```python
from build123d import *

# Parameters (mm, degrees)
BOSS_EXTRUDE1_DEPTH = 13
BOSS_EXTRUDE2_DEPTH = 2.5
SKETCH3_R           = 7
BOSS_EXTRUDE3_DEPTH = 5


with BuildPart() as part:
    # Sketch1 → Boss-Extrude1 (new body)
    with BuildSketch(Plane(origin=(0, 0, 0), x_dir=(1, 0, 0), z_dir=(0, 1, 0))):
        with BuildLine():
            ThreePointArc((5.85, 0), (5.148142373, 2.778332254), (3.210981158, 4.89))
            Line((3.210981158, 4.89), (-3.210981158, 4.89))
            ThreePointArc((-3.210981158, 4.89), (-5.148142373, 2.778332254), (-5.85, 0))
            Line((-5.85, 0), (5.85, 0))
        make_face()
        with BuildLine():
            ThreePointArc((3.210981158, -4.89), (5.148142373, -2.778332254), (5.85, 0))
            Line((5.85, 0), (-5.85, 0))
            ThreePointArc((-5.85, 0), (-5.148142373, -2.778332254), (-3.210981158, -4.89))
            Line((-3.210981158, -4.89), (3.210981158, -4.89))
        make_face()
    extrude(amount=BOSS_EXTRUDE1_DEPTH)

    # Sketch2 → Boss-Extrude2 (add)
    with BuildSketch(Plane(origin=(0, 13, 0), x_dir=(1, 0, 0), z_dir=(0, 1, 0))):
        with BuildLine():
            Line((0, 4.89), (0, 7.75))
            ThreePointArc((0, 7.75), (-4.510404638, 6.302281333), (-7.335700376, 2.5))
            ThreePointArc((-7.335700376, 2.5), (-7.75, 0), (-7.335700376, -2.5))
            ThreePointArc((-7.335700376, -2.5), (-4.510404638, -6.302281333), (0, -7.75))
            Line((0, -7.75), (0, -4.89))
            Line((0, -4.89), (-3.210981158, -4.89))
            ThreePointArc((-3.210981158, -4.89), (-5.85, 0), (-3.210981158, 4.89))
            Line((-3.210981158, 4.89), (0, 4.89))
        make_face()
        with BuildLine():
            ThreePointArc((7.335700376, 2.5), (4.510404638, 6.302281333), (0, 7.75))
            Line((0, 7.75), (0, 4.89))
            Line((0, 4.89), (3.210981158, 4.89))
            ThreePointArc((3.210981158, 4.89), (5.85, 0), (3.210981158, -4.89))
            Line((3.210981158, -4.89), (0, -4.89))
            Line((0, -4.89), (0, -7.75))
            ThreePointArc((0, -7.75), (4.510404638, -6.302281333), (7.335700376, -2.5))
            ThreePointArc((7.335700376, -2.5), (7.645723573, -1.267048162), (7.75, 0))
            ThreePointArc((7.75, 0), (7.645723573, 1.267048162), (7.335700376, 2.5))
        make_face()
        with BuildLine():
            Line((3.210981158, 4.89), (0, 4.89))
            Line((0, 4.89), (0, -4.89))
            Line((0, -4.89), (3.210981158, -4.89))
            ThreePointArc((3.210981158, -4.89), (5.85, 0), (3.210981158, 4.89))
        make_face()
        with BuildLine():
            Line((9.835700376, 2.5), (7.335700376, 2.5))
            ThreePointArc((7.335700376, 2.5), (7.645723573, 1.267048162), (7.75, 0))
            ThreePointArc((7.75, 0), (7.645723573, -1.267048162), (7.335700376, -2.5))
            Line((7.335700376, -2.5), (9.835700376, -2.5))
            Line((9.835700376, -2.5), (9.835700376, 2.5))
        make_face()
        with BuildLine():
            Line((0, -4.89), (0, 4.89))
            Line((0, 4.89), (-3.210981158, 4.89))
            ThreePointArc((-3.210981158, 4.89), (-5.85, 0), (-3.210981158, -4.89))
            Line((-3.210981158, -4.89), (0, -4.89))
        make_face()
        with BuildLine():
            ThreePointArc((-7.335700376, -2.5), (-7.75, 0), (-7.335700376, 2.5))
            Line((-7.335700376, 2.5), (-9.835700376, 2.5))
            Line((-9.835700376, 2.5), (-9.835700376, -2.5))
            Line((-9.835700376, -2.5), (-7.335700376, -2.5))
        make_face()
    extrude(amount=BOSS_EXTRUDE2_DEPTH)

    # Sketch3 → Boss-Extrude3 (add)
    with BuildSketch(Plane(origin=(0, 15.5, 0), x_dir=(1, 0, 0), z_dir=(0, 1, 0))):
        Circle(SKETCH3_R)
        with BuildLine():
            ThreePointArc((-6.837397166, -1.5), (-7, 0), (-6.837397166, 1.5))
            Line((-6.837397166, 1.5), (-8.837397166, 1.5))
            Line((-8.837397166, 1.5), (-8.837397166, -1.5))
            Line((-8.837397166, -1.5), (-6.837397166, -1.5))
        make_face()
        with BuildLine():
            Line((8.837397166, 1.5), (6.837397166, 1.5))
            ThreePointArc((6.837397166, 1.5), (6.959230567, 0.754393744), (7, 0))
            ThreePointArc((7, 0), (6.959230567, -0.754393744), (6.837397166, -1.5))
            Line((6.837397166, -1.5), (8.837397166, -1.5))
            Line((8.837397166, -1.5), (8.837397166, 1.5))
        make_face()
    extrude(amount=BOSS_EXTRUDE3_DEPTH)


solid = part.part
```
Work out the finished part from the listing and answer in its coordinate system (mm). A direction names the side the tool comes from. Round coordinates to 2 decimals unless told otherwise and drop trailing zeros. Loops run counter-clockwise (first coordinate to the right, second up) from the corner with the lowest first, then second, coordinate; pieces in that order, holes last. Notation, with made-up numbers: M 88,-26 L 126,-26 A17 cw 126,-1 Z; hole C -25.5,-34.75 d11. An arc over 180 degrees is marked long. One line per question, with ' | ' between items.
Q1. Each of these flat-tipped pins is pushed along its axis until it touches: pin 1 Ø1.5 at (y, z) = (18, 0) entering from +X; pin 2 Ø1 at (x, z) = (4, 0.5) entering from -Y; pin 3 Ø1.2 at (x, y) = (-9, 14.5) entering from +Z; pin 4 Ø0.8 at (x, y) = (-8, 14.5) entering from -Z. Where does it stop, or does it pass through?
Conclusion:
pin 1: stops at x = 8.84 | pin 2: stops at y = 0 | pin 3: stops at z = 2.5 | pin 4: stops at z = -2.5
Q2. Find section D-D, the plane y = 10.25. Give the vertices of the cut face in (x, z), then the cut area to 3 significant figures.
Conclusion:
outline: M -3.21,-4.89 L 3.21,-4.89 A5.85 ccw 3.21,4.89 L -3.21,4.89 A5.85 ccw Z | area: 99.1 mm2
Q3. Find section B-B, the plane y = 14. Give the vertices of the cut face in (x, z).
Conclusion:
outline: M -9.84,-2.5 L -7.34,-2.5 A7.75 ccw 7.34,-2.5 L 9.84,-2.5 L 9.84,2.5 L 7.34,2.5 A7.75 ccw -7.34,2.5 L -9.84,2.5 Z
Q4. A tool of negligible diameter and unlimited length cuts with its end or side. For faces 1 (the flat face through (-8.837, 18, 0)), 2 (the flat face through (-9, 14, -2.5)), 3 (the flat face through (0, 6, 4.89)), 4 (the flat face through (-9, 14, 2.5)), 5 (the flat face through (0, 6, -4.89)), from which of +Z, -Z, +X, -X, +Y, -Y can it reach the whole face along a straight path? Write none if from no direction.
Conclusion:
face 1: +Z, -Z, -X, +Y | face 2: -Z, -X, +Y, -Y | face 3: +Z, +X, -X, -Y | face 4: +Z, -X, +Y, -Y | face 5: -Z, +X, -X, -Y
Q5. Find section C-C, the plane z = 4. Give the vertices of the cut face in (x, y).
Conclusion:
outline: M -6.64,13 L -4.27,13 L -4.27,0 L 4.27,0 L 4.27,13 L 6.64,13 L 6.64,15.5 L 5.74,15.5 L 5.74,20.5 L -5.74,20.5 L -5.74,15.5 L -6.64,15.5 Z
Q6. Find section A-A, the plane x = -2.25. Give the vertices of the cut face in (y, z).
Conclusion:
outline: M 0,-4.89 L 13,-4.89 L 13,-7.42 L 15.5,-7.42 L 15.5,-6.63 L 20.5,-6.63 L 20.5,6.63 L 15.5,6.63 L 15.5,7.42 L 13,7.42 L 13,4.89 L 0,4.89 Z
Q7. Consider line 1 along Z through (x, y) = (1.5, 12.5); line 2 along Z through (x, y) = (-7.5, 17.75); line 3 along Y through (x, z) = (-3.25, -5.75). Determine where each line is inside the solid, lowest interval first. Write a range as from..to.
Conclusion:
line 1: z = -4.89..4.89 | line 2: z = -1.5..1.5 | line 3: y = 13..20.5
